Work out the finished part from the listing and answer in its coordinate system (mm). A direction names the side the tool comes from. Coordinates: 2 decimals unless noted, no trailing zeros. Order: outer loops, then holes, each group sorted by start corner. A loop starts at its lowest first (then second) coordinate and runs counter-clockwise, first axis right, second up.
```python
from build123d import *

# Parameters (mm, degrees)
ESQUISSE1_W             = 18
ESQUISSE1_H             = 11
ESQUISSE1_R             = 1.5
BOSS_EXTRU_1_DEPTH      = 3
ESQUISSE2_W             = 18
ESQUISSE2_H             = 3
BOSS_EXTRU_2_DEPTH      = 5
ESQUISSE3_W             = 3
ESQUISSE3_H             = 5
BOSS_EXTRU_3_DEPTH      = 18
ESQUISSE4_R             = 0.5
ESQUISSE4_R_2           = 1
ENL_V_MAT_EXTRU_1_DEPTH = 18


with BuildPart() as part:
    # Esquisse1 → Boss.-Extru.1 (new body)
    with BuildSketch(Plane.XY):
        with Locations((-8.232718894, -0.823732719)):
            Rectangle(ESQUISSE1_W, ESQUISSE1_H)
        with Locations((-14.232718894, -2.323732719)):
            Circle(ESQUISSE1_R, mode=Mode.SUBTRACT)
        with Locations((-2.232718894, -2.323732719)):
            Circle(ESQUISSE1_R, mode=Mode.SUBTRACT)
    extrude(amount=BOSS_EXTRU_1_DEPTH)

    # Esquisse2 → Boss.-Extru.2 (add)
    with BuildSketch(Plane.XY.offset(3)):
        with Locations((-8.232718894, 3.176267281)):
            Rectangle(ESQUISSE2_W, ESQUISSE2_H)
    extrude(amount=BOSS_EXTRU_2_DEPTH)

    # Esquisse3 → Boss.-Extru.3 (add)
    with BuildSketch(Plane(origin=(0, 4.676267281, 0), x_dir=(1, 0, 0), z_dir=(0, 1, 0))):
        with Locations((-8.232718894, -4)):
            Rectangle(ESQUISSE3_W, ESQUISSE3_H)
    extrude(amount=BOSS_EXTRU_3_DEPTH)

    # Esquisse4 → Enlèv. mat.-Extru.1 (cut)
    with BuildSketch(Plane(origin=(-6.732718894, 0, 0), x_dir=(0, 0, -1), z_dir=(1, 0, 0))):
        with BuildLine():
            ThreePointArc((-4, 7.176267281), (-4.5, 6.676267281), (-4, 6.176267281))
            Line((-4, 6.176267281), (-4, 7.176267281))
        make_face()
        with BuildLine():
            Line((-4, 7.176267281), (-4, 6.176267281))
            ThreePointArc((-4, 6.176267281), (-3.646446609, 6.322713891), (-3.5, 6.676267281))
            ThreePointArc((-3.5, 6.676267281), (-3.646446609, 7.029820672), (-4, 7.176267281))
        make_face()
        with Locations((-4, 8.676267281)):
            Circle(ESQUISSE4_R)
        with Locations((-4, 10.676267281)):
            Circle(ESQUISSE4_R)
        with Locations((-4, 12.676267281)):
            Circle(ESQUISSE4_R)
        with Locations((-4, 14.676267281)):
            Circle(ESQUISSE4_R)
        with Locations((-4, 16.676267281)):
            Circle(ESQUISSE4_R)
        with Locations((-4, 21.176267281)):
            Circle(ESQUISSE4_R_2)
    extrude(amount=-ENL_V_MAT_EXTRU_1_DEPTH, mode=Mode.SUBTRACT)


solid = part.part
```
1. The part is cut by section A-A (x = -9). Determine the outline of the cut face in (y, z), plus the area to 3 significant figures.
2. The part is cut by section B-B (y = 11.5). Determine the outline of the cut face in (x, z), plus the area to 3 significant figures.
3. Consider probe 1 along Y at (x, z) = (0.25, 5); probe 2 along Z at (x, y) = (-10.25, -2.75); probe 3 along X at (y, z) = (14.25, 3.5). Determine where each line is inside the solid, lowest interval first.
4. Flat-ended cylindrical pins translate along their axes: pin 1 (3 mm diameter, centred on y = 21.18, z = 4, fed in from +X); pin 2 (6 mm diameter, centred on x = -10, y = 16.5, fed in from +Z); pin 3 (2.5 mm diameter, centred on x = -8.5, y = 11.5, fed in from -Z). Find the tip coordinate at first contact, or state that the pin passes through.
5. The mould has two halves that part along Z. Classify faces 1 (the flat face through (-8, 14, 6.5)), 2 (the flat face through (-8, 1.676, 5)), 3 (the cylindrical face through (-8.21, 13.17, 4.07)), 4 (the cylindrical face through (-8.21, 16.19, 4.11)): released by +Z, released by -Z, zero draft, split by the parting line, or undercut.
6. The part is cut by section C-C (x = -5). Determine the outline of the cut face in (y, z).
7. For faces 5 (the flat face through (-6.733, 14, 4)), 6 (the flat face through (-9.733, 14, 4)), 7 (the flat face through (-8, 14, 1.5)), 8 (the flat face through (-8, -2, 3)), determine the directions among +Z, -Z, +X, -X, +Y, -Y from which every point of the face is accessible in a straight line to the end or side of a thin tool.
Worked out:
1. outline: (-6.32, 0) - (4.68, 0) - (4.68, 1.5) - (22.68, 1.5) - (22.68, 6.5) - (4.68, 6.5) - (4.68, 8) - (1.68, 8) - (1.68, 3) - (-6.32, 3) - close; hole circle Ø1 at (6.68, 4); hole circle Ø1 at (8.68, 4); hole circle Ø1 at (10.68, 4); hole circle Ø1 at (12.68, 4); hole circle Ø1 at (14.68, 4); hole circle Ø1 at (16.68, 4); hole circle Ø2 at (21.18, 4)
1. area: 130 mm2
2. outline: (-9.73, 1.5) - (-6.73, 1.5) - (-6.73, 6.5) - (-9.73, 6.5) - close
2. area: 15.0 mm2
3. probe 1: y = 1.68 to 4.68
3. probe 2: z = 0 to 3
3. probe 3: x = -9.73 to -6.73
4. pin 1: stops at x = -6.73
4. pin 2: stops at z = 6.5
4. pin 3: stops at z = 1.5
5. face 1: released by +Z
5. face 2: zero draft
5. face 3: undercut
5. face 4: undercut
6. outline: (-6.32, 0) - (4.68, 0) - (4.68, 8) - (1.68, 8) - (1.68, 3) - (-6.32, 3) - close
7. face 5: +Z, -Z, +X, +Y
7. face 6: +Z, -Z, -X, +Y
7. face 7: -Z, +X, -X, +Y
7. face 8: +Z, +X, -X, -Y
